The listing builds one solid part. Answer for the finished solid, in the listing's coordinates (mm). Face numbers are marked on the shaded views. A direction names the side the tool comes from. Coordinates: 2 decimals unless noted, no trailing zeros. Write each loop counter-clockwise with the first axis right and the second up, starting at its lowest first coordinate (ties: lowest second). Pieces come first, ordered by that corner, then holes. Notation, with made-up numbers: M -14,76 L 17,76 A14 cw 17,87 Z; hole C 34.25,12.5 d11. An arc over 180 degrees is marked long. Answer as CSV lines item,"result".
```python
from build123d import *
from build123d.topology import SkipClean

# Parameters (mm, degrees)
SKETCH1_R               = 6
SKETCH1_R_2             = 1.5
BOSS_EXTRUDE1_DEPTH     = 75
SKETCH2_R               = 1.5
CUT_EXTRUDE1_DEPTH      = 75
BOSS_EXTRUDE2_START     = 10
SKETCH4_R               = 6
SKETCH4_R_2             = 1.5
BOSS_EXTRUDE2_DEPTH     = 10
SKETCH5_W               = 4
SKETCH5_H               = 27.545605052
CUT_EXTRUDE2_DEPTH      = 17
CUT_EXTRUDE4_DEPTH      = 15
CUT_EXTRUDE4_DEPTH_BACK = 15
SKETCH7_R               = 3
SKETCH8_R               = 3
CUT_EXTRUDE5_DEPTH      = 14


with BuildPart() as part:
    # Sketch1 → Boss-Extrude1 (new body)
    with BuildSketch(Plane(origin=(0, 0, 0), x_dir=(1, 0, 0), z_dir=(0, 1, 0))):
        with Locations(Location((0, 0, 0), (0, 0, 270))):
            Circle(SKETCH1_R)
        with Locations(Location((0, 0, 0), (0, 0, 270))):
            Circle(SKETCH1_R_2, mode=Mode.SUBTRACT)
    extrude(amount=BOSS_EXTRUDE1_DEPTH)

    # Sketch2 → Cut-Extrude1 (cut)
    with BuildSketch(Plane.XY):
        with Locations((0, 23.5)):
            Circle(SKETCH2_R)
        with Locations((0, 54)):
            Circle(SKETCH2_R)
    extrude(amount=-CUT_EXTRUDE1_DEPTH, mode=Mode.SUBTRACT)

    # Sketch4 → Boss-Extrude2 (add)
    with BuildSketch(Plane.XZ.offset(BOSS_EXTRUDE2_START)):
        with Locations(Location((0, 0, 0), (0, 0, 270))):
            Circle(SKETCH4_R)
        with Locations(Location((0, 0, 0), (0, 0, 270))):
            Circle(SKETCH4_R_2, mode=Mode.SUBTRACT)
    extrude(amount=-BOSS_EXTRUDE2_DEPTH)

    # Sketch5 → Cut-Extrude2 (cut)
    with SkipClean():  # the faces are left unmerged after this step: merging them gives an invalid solid
        with BuildSketch(Plane.XZ.offset(10)):
            Rectangle(SKETCH5_W, SKETCH5_H)
        extrude(amount=-CUT_EXTRUDE2_DEPTH, mode=Mode.SUBTRACT)

    # Sketch7 → Cut-Extrude4 (cut, two sides: drawn at the far end of the back side and taken through both)
    with SkipClean():  # the faces are left unmerged after this step: merging them gives an invalid solid
        with BuildSketch(Plane(origin=(-2, 0, 0), x_dir=(0, 0, -1), z_dir=(1, 0, 0)).offset(-CUT_EXTRUDE4_DEPTH_BACK)):
            with Locations(Location((0, -2, 0), (0, 0, 180))):
                Circle(SKETCH7_R)
        extrude(amount=CUT_EXTRUDE4_DEPTH + CUT_EXTRUDE4_DEPTH_BACK, mode=Mode.SUBTRACT)

    # Sketch8 → Cut-Extrude5 (cut)
    with SkipClean():  # the faces are left unmerged after this step: merging them gives an invalid solid
        with BuildSketch(Plane(origin=(0, 75, 0), x_dir=(1, 0, 0), z_dir=(0, 1, 0))):
            with Locations(Location((0, 0, 0), (0, 0, 270))):
                Circle(SKETCH8_R)
        extrude(amount=-CUT_EXTRUDE5_DEPTH, mode=Mode.SUBTRACT)


solid = part.part
```
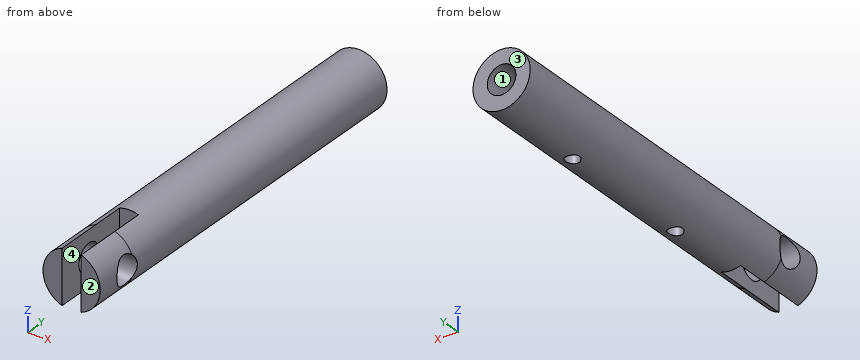
Q1. Flat-ended cylindrical pins translate along their axes: pin 1 Ø5 at (x, z) = (0, 0) entering from +Y; pin 2 Ø5 at (x, y) = (2.5, 9.5) entering from -Z; pin 3 Ø1.2 at (x, z) = (0.5, -2.5) entering from -Y; pin 4 Ø2.5 at (x, z) = (0, 0) entering from -Y. Find the tip coordinate at first contact, or state that the pin passes through.
Output:
pin 1,"y = 61"
pin 2,"z = -6"
pin 3,"y = 7"
pin 4,"through"
Q2. The mould has two halves that part along X. Classify the marked faces 1 and 2: pulls with the +X half, pulls with the -X half, needs draft (parallel to the pull), parting line crosses it, or undercut.
Output:
face 1,"undercut"
face 2,"needs draft"
Q3. For the marked faces 3 and 4, determine the directions among +Z, -Z, +X, -X, +Y, -Y from which every point of the face is accessible in a straight line to the end or side of a thin tool.
Output:
face 3,"+Z, -Z, +X, -X, +Y"
face 4,"+Z, -Z, -Y"
Q4. Find section B-B (y = 14). Give the vertices of the cut face in (x, z), and give its area (3 significant figures).
Output:
outline,"C 0,0 d12; hole C 0,0 d3"
area,"106 mm2"
Q5. Find section D-D (x = 4.5). Give the vertices of the cut face in (y, z), and give its area (3 significant figures).
Output:
outline,"M -10,-3.97 L 75,-3.97 L 75,3.97 L -10,3.97 Z; hole C -2,0 d6"
area,"646 mm2"
Q6. Straight lines are drawn through the part: line 1 (Y direction, x = 0, z = -2); line 2 (Z direction, x = 0, y = 27); line 3 (Y direction, x = -0.5, z = -4.25). For each, find the intervals that lie inside material, in ascending order.
Output:
line 1,"7 to 22, 25 to 52.5, 55.5 to 61"
line 2,"-6 to -1.5, 1.5 to 6"
line 3,"7 to 22.09, 24.91 to 52.59, 55.41 to 75"
Q7. Find section C-C (x = -4.25). Give the vertices of the cut face in (y, z).
Output:
outline,"M -10,-4.24 L 75,-4.24 L 75,4.24 L -10,4.24 Z; hole C -2,0 d6"
Q8. Find section A-A (y = -2). Give the vertices of the cut face in (x, z).
Output:
outline,"M -5.2,-3 A6 ccw -2,-5.66 L -2,-3 Z; M -5.2,3 L -2,3 L -2,5.66 A6 ccw Z; M 2,-5.66 A6 ccw 5.2,-3 L 2,-3 Z; M 2,3 L 5.2,3 A6 ccw 2,5.66 Z"
